Build history of the part. All positions in model axes, mm. A direction names the side the tool comes from. Give positions to 0.01 mm unless a question says otherwise; leave off trailing zeros. Write each loop counter-clockwise with the first axis right and the second up, starting at its lowest first coordinate (ties: lowest second). Pieces come first, ordered by that corner, then holes.
from build123d import *

# Parameters (mm, degrees)
BOSS_EXTRUDE1_DEPTH = 3.175
BOSS_EXTRUDE2_DEPTH = 3.175
CUT_EXTRUDE2_DEPTH  = 113.944871324
CIRPATTERN1_COUNT   = 6


with BuildPart() as part:
    # Sketch1 → Boss-Extrude1 (new body)
    with BuildSketch(Plane(origin=(0, 0, 0), x_dir=(1, 0, 0), z_dir=(0, 1, 0))):
        Polygon((-39.375288359, 68.2), (-78.750576717, 0), (-39.375288359, -68.2), (39.375288359, -68.2), (78.750576717, 0), (39.375288359, 68.2), align=None)
    extrude(amount=BOSS_EXTRUDE1_DEPTH)

    # Sketch2 → Boss-Extrude2 (add)
    with BuildSketch(Plane(origin=(0, 0, 0), x_dir=(1, 0, 0), z_dir=(0, 1, 0))):
        with BuildLine():
            ThreePointArc((16.512644179, 74.55), (16.887402094, 70.393871043), (13.337644179, 68.2))
            Line((13.337644179, 68.2), (26.037644179, 68.2))
            ThreePointArc((26.037644179, 68.2), (22.487886265, 70.393871043), (22.862644179, 74.55))
            ThreePointArc((22.862644179, 74.55), (23.237402094, 78.706128957), (19.687644179, 80.9))
            ThreePointArc((19.687644179, 80.9), (16.137886265, 78.706128957), (16.512644179, 74.55))
        make_face()
    boss_extrude2 = extrude(amount=BOSS_EXTRUDE2_DEPTH)

    # Sketch2<3> → Cut-Extrude2 (cut, through all)
    with BuildSketch(Plane(origin=(0, 0, 0), x_dir=(1, 0, 0), z_dir=(0, 1, 0))):
        with BuildLine():
            Line((-13.337644179, 68.2), (-26.037644179, 68.2))
            ThreePointArc((-26.037644179, 68.2), (-22.487886265, 66.006128957), (-22.862644179, 61.85))
            ThreePointArc((-22.862644179, 61.85), (-23.237402094, 57.693871043), (-19.687644179, 55.5))
            ThreePointArc((-19.687644179, 55.5), (-16.137886265, 57.693871043), (-16.512644179, 61.85))
            ThreePointArc((-16.512644179, 61.85), (-16.887402094, 66.006128957), (-13.337644179, 68.2))
        make_face()
    cut_extrude2 = extrude(amount=CUT_EXTRUDE2_DEPTH, mode=Mode.SUBTRACT)

    # CirPattern1: Boss-Extrude2, Cut-Extrude2 ×6 about axis
    cirpattern1_axis = Axis((0, 0, 0), (0, 1, 0))
    add([boss_extrude2.rotate(cirpattern1_axis, i * 360 / CIRPATTERN1_COUNT) for i in range(1, CIRPATTERN1_COUNT)])
    add([cut_extrude2.rotate(cirpattern1_axis, i * 360 / CIRPATTERN1_COUNT) for i in range(1, CIRPATTERN1_COUNT)], mode=Mode.SUBTRACT)


solid = part.part
1. Mould opens along Z. For faces 4 (the face through (75.369, 1.565, 5.856)), 5 (the face through (75.463, 1.565, -5.695)), 6 (the face through (59.156, 1.565, -33.938)) say: pulls with the +Z half, pulls with the -Z half, needs draft (parallel to the pull), parting line crosses it, or undercut.
2. Saw through at B-B on z = -32. Give the cut face in (x, y) (3 decimals), plus the area to 3 significant figures.
3. Drop flat-ended pins along their axis: pin 1 (1 mm diameter, centred on x = -35, y = 1, fed in from +Z); pin 2 (1.5 mm diameter, centred on y = 1.5, z = -61.5, fed in from +X). Give the stop position or say it passes through.
4. Drill centre lines: line 1 along Z through (x, y) = (59, 0.4); line 2 along Z through (x, y) = (-29, 1.65); line 3 along X through (y, z) = (2.55, -10). Where is each one in solid material? Low to high.
5. Saw through at A-A on x = -29. Give the cut face in (y, z) (3 decimals).
6. 3-axis set-ups, long thin cutter, end or side, ignore diameter. For faces 1 (the face through (58.97, 1.57, 34.26)), 2 (the face through (-58.97, 1.57, -34.26)), 3 (the face through (42.66, 1.57, 62.51)): which of +Z, -Z, +X, -X, +Y, -Y reach the whole face in a straight line?
Outcome:
1. face 4: pulls with the +Z half
1. face 5: undercut
1. face 6: pulls with the -Z half
2. outline: (-60.275, 0) - (60.275, 0) - (60.275, 3.175) - (-60.275, 3.175) - close
2. area: 383 mm2
3. pin 1: stops at z = 68.2
3. pin 2: stops at x = 43.68
4. line 1: z = -34.21 to 9.48, 15.89 to 34.21, 52.23 to 58.81
4. line 2: z = -68.2 to 68.2
4. line 3: x = -72.98 to -64.27, -58.42 to 72.98
5. outline: (0, -68.2) - (3.175, -68.2) - (3.175, 68.2) - (0, 68.2) - close
6. face 1: +X, +Y, -Y
6. face 2: -X, +Y, -Y
6. face 3: +Z, +Y, -Y
